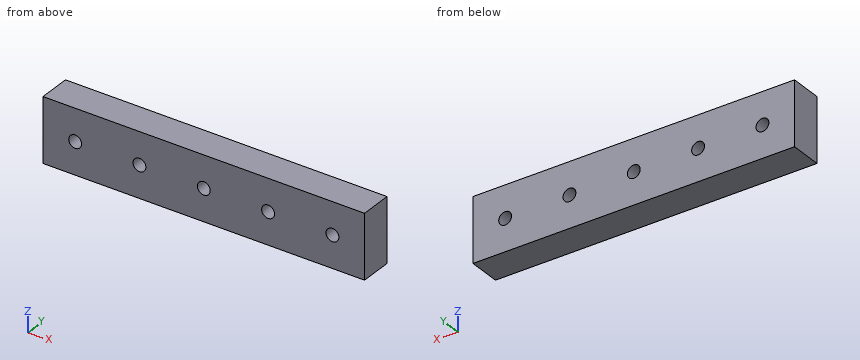
Autodesk Inventor part; units mm, degrees
ref_plane "YZ Plane" through (0, 0, 0) normal (1, 0, 0) x (0, 1, 0)
ref_plane "XZ Plane" through (0, 0, 0) normal (0, 1, 0) x (-1, 0, 0)
ref_plane "XY Plane" through (0, 0, 0) normal (0, 0, 1) x (1, 0, 0)
sketch "Skizze1" plane through (0, 0, 0) normal (0, 1, 0) x (-1, 0, 0)
  line L0 (-50, 10) -> (50, 10)
  line L1 (50, 10) -> (50, -10)
  line L2 (50, -10) -> (-50, -10)
  line L3 (-50, -10) -> (-50, 10)
  line L4 (-50, 10) -> (50, -10) construction
  line L5 (50, 10) -> (-50, -10) construction
  point P0 (0, 0)
  dimension "d0" = 100
  dimension "d1" = 20
extrude "Extrusion1" add sketch "Skizze1" along normal blind 10
sketch "Skizze2" plane through (0, 10, 0) normal (0, 1, 0) x (1, 0, 0)
  line L0 (-70, 0) -> (70, 0)
  line L1 (-50, 10) -> (-50, -10)
  point P0 (0, 0)
  point P1 (-40, 0)
  point P2 (-20, 0)
  point P3 (0, 0)
  point P4 (20, 0)
  point P5 (40, 0)
  dimension "d4" = 10
  dimension "d7" = 20
hole "Bohrung1" at (-40, 10, 0) at (-20, 10, 0) at (0, 10, 0) at (20, 10, 0) at (40, 10, 0) direction (0, -1, 0) diameter 4 end through all
properties part number "Linear_rail"
Geometry check sheet. Reference: the model listing, model coordinates, mm. Give positions to 0.01 mm unless a question says otherwise; leave off trailing zeros. Loops run counter-clockwise (first coordinate to the right, second up) from the corner with the lowest first, then second, coordinate; pieces in that order, holes last. Notation, with made-up numbers: M 64,78 L 70,78 A33 cw 70,113 Z; hole C -27,-22.5 d6. An arc over 180 degrees is marked long. Answer as CSV lines item,"result".
Item 1: Material ranges on line 1 (X direction, y = 6.5, z = 0.25); line 2 (Z direction, x = -20, y = 3.75); line 3 (X direction, y = 2.25, z = 1.5), recorded low to high.
Values:
line 1,"x = -50 to -41.98, -38.02 to -21.98, -18.02 to -1.98, 1.98 to 18.02, 21.98 to 38.02, 41.98 to 50"
line 2,"z = -10 to -2, 2 to 10"
line 3,"x = -50 to -41.32, -38.68 to -21.32, -18.68 to -1.32, 1.32 to 18.68, 21.32 to 38.68, 41.32 to 50"
Item 2: Cross-section at A-A on x = -40. Record the cut outline in (y, z), and give its area (3 significant figures).
Values:
outline,"M 0,-10 L 10,-10 L 10,-2 L 0,-2 Z; M 0,2 L 10,2 L 10,10 L 0,10 Z"
area,"160 mm²"
Item 3: Cross-section at C-C on z = 0. Record the cut outline in (x, y), and give its area (3 significant figures).
Values:
outline,"M -50,0 L -42,0 L -42,10 L -50,10 Z; M -38,0 L -22,0 L -22,10 L -38,10 Z; M -18,0 L -2,0 L -2,10 L -18,10 Z; M 2,0 L 18,0 L 18,10 L 2,10 Z; M 22,0 L 38,0 L 38,10 L 22,10 Z; M 42,0 L 50,0 L 50,10 L 42,10 Z"
area,"800 mm²"
Item 4: Cross-section at B-B on y = 5. Record the cut outline in (x, z), and give its area (3 significant figures).
Values:
outline,"M -50,-10 L 50,-10 L 50,10 L -50,10 Z; hole C -40,0 d4; hole C -20,0 d4; hole C 0,0 d4; hole C 20,0 d4; hole C 40,0 d4"
area,"1,940 mm²"
